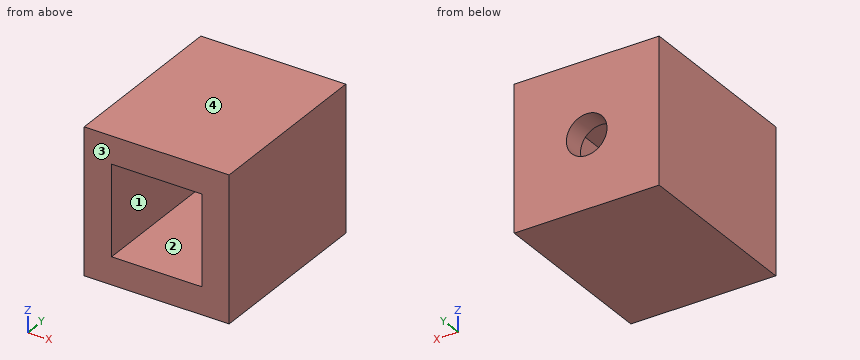
Autodesk Inventor part; units mm, degrees
ref_plane "YZ Plane" through (0, 0, 0) normal (1, 0, 0) x (0, 1, 0)
ref_plane "XZ Plane" through (0, 0, 0) normal (0, 1, 0) x (-1, 0, 0)
ref_plane "XY Plane" through (0, 0, 0) normal (0, 0, 1) x (1, 0, 0)
sketch "Sketch1" plane through (0, 0, 0) normal (0, 1, 0) x (-1, 0, 0)
  line L0 (0, 0) -> (-7.7978, 0)
  line L1 (-7.7978, 0) -> (-7.7978, -7.7978)
  line L2 (-7.7978, -7.7978) -> (0, -7.7978)
  line L3 (0, -7.7978) -> (0, 0)
  dimension "d0" = 7.7978
  dimension "d1" = 7.7978
extrude "Extrusion1" add sketch "Sketch1" along normal blind 9.6088
shell "Shell1" thickness 1.4732 removed faces 1 at (5.1985, 0, -2.5993)
sketch "Sketch2" plane through (1.4732, 8.1356, -1.4732) normal (0, -1, 0) x (1, 0, 0)
  line L0 (0, -4.8514) -> (0, 0)
  line L1 (4.8514, 0) -> (4.8514, -4.8514)
  line L2 (0, 0) -> (4.8514, 0)
  line L3 (4.8514, 0) -> (4.8514, -4.8514)
  line L4 (4.8514, -4.8514) -> (0, -4.8514)
  line L5 (0, -4.8514) -> (0, 0)
  point P0 (-1.4732, 1.4732)
extrude "Extrusion2" cut sketch "Sketch2" against normal blind 0.3048
sketch "Sketch3" plane through (1.4732, 8.4404, -1.4732) normal (0, -1, 0) x (1, 0, 0)
  line L0 (0, 0) -> (4.8514, 0) construction
  line L1 (4.8514, 0) -> (4.8514, -4.8514) construction
  line L2 (4.8514, -4.8514) -> (0, -4.8514) construction
  line L3 (0, -4.8514) -> (0, 0) construction
  line L4 (0, -4.8514) -> (0, 0) construction
  line L5 (0, -2.4257) -> (4.8514, -2.4257) construction
  line L6 (0, 0) -> (4.8514, 0) construction
  line L7 (2.4257, 0) -> (2.4257, -4.8514) construction
  circle A0 centre (2.4257, -2.4257) radius 1.0935
  point P0 (-1.4732, 1.4732)
  dimension "d7" = 2.1869
extrude "Extrusion3" cut sketch "Sketch3" against normal blind 1.27
properties part number "Sample 1x1 tall" material "ABS Plastic"
Could you check a few things on this model? Use its own coordinates, in mm. Face numbers are marked on the shaded views. Give positions to 0.01 mm unless a question says otherwise; leave off trailing zeros. Loops run counter-clockwise (first coordinate to the right, second up) from the corner with the lowest first, then second, coordinate; pieces in that order, holes last. Notation, with made-up numbers: (85.25, 2) - (107.25, 2) arc R27 ccw to (107.25, 20) - close; hole circle Ø3 at (9.5, -1.75). An arc over 180 degrees is marked (long way). Use one line per item in the form item = value.
1. I need wall thicknesses on probe 1 along X at (y, z) = (3, -6.25); probe 2 along Z at (x, y) = (5.75, 4); probe 3 along Y at (x, z) = (6, -2.75). Which ranges of each line are inside material? Lowest first, please.
Response values:
probe_1 = 0 to 1.47, 6.32 to 7.8
probe_2 = -7.8 to -6.32, -1.47 to 0
probe_3 = 8.44 to 9.61
2. I want a section at D-D (z = -2). Please give me the cut outline in (x, y), and give its area (3 significant figures).
Response values:
outline = (0, 0) - (1.47, 0) - (1.47, 8.44) - (6.32, 8.44) - (6.32, 0) - (7.8, 0) - (7.8, 9.61) - (0, 9.61) - close
area = 34.0 mm²
3. I want a section at C-C (x = 4.75). Please give me the cut outline in (y, z).
Response values:
outline = (0, -7.8) - (9.61, -7.8) - (9.61, -4.59) - (8.44, -4.59) - (8.44, -6.32) - (0, -6.32) - close; (0, -1.47) - (8.44, -1.47) - (8.44, -3.21) - (9.61, -3.21) - (9.61, 0) - (0, 0) - close
4. I'm going to push a flat-ended pin straight in: pin 1 Ø1.5 at (x, z) = (4, -5) entering from -Y. Where does the tip first touch, or does it pass through?
Response values:
pin_1 = 8.44
5. I want a section at A-A (y = 3.75). Please give me the cut outline in (x, z).
Response values:
outline = (0, -7.8) - (7.8, -7.8) - (7.8, 0) - (0, 0) - close; hole (1.47, -6.32) - (6.32, -6.32) - (6.32, -1.47) - (1.47, -1.47) - close
6. I want a section at B-B (z = -4.5). Please give me the cut outline in (x, y), and give its area (3 significant figures).
Response values:
outline = (0, 0) - (1.47, 0) - (1.47, 8.44) - (2.99, 8.44) - (2.99, 9.61) - (0, 9.61) - close; (4.81, 8.44) - (6.32, 8.44) - (6.32, 0) - (7.8, 0) - (7.8, 9.61) - (4.81, 9.61) - close
area = 31.8 mm²
7. Thinking about a two-plate mould opening in Z: for the marked faces 1, 2, 3 and 4, which applies, released by +Z, released by -Z, zero draft, split by the parting line, or undercut?
Response values:
face_1 = undercut
face_2 = undercut
face_3 = zero draft
face_4 = released by +Z
